from build123d import *
from build123d.topology import SkipClean

# Parameters (mm, degrees)
SKETCH_1_R               = 25
EXTRUDE_1_DEPTH          = 8
SKETCH_2_R               = 3
EXTRUDE_2_DEPTH          = 10
EXTRUDE_START            = 10
SKETCH_3_R               = 25
SKETCH_3_R_2             = 20
EXTRUDE_3_DEPTH          = 10
SKETCH_4_R               = 5
EXTRUDE_4_DEPTH          = 2
SKETCH_5_R               = 2.5
EXTRUDE_5_DEPTH          = 8
EXTRUDE_START_2          = 5
SKETCH_6_R               = 25
SKETCH_6_R_2             = 5
EXTRUDE_6_DEPTH          = 5
CUT_EXTRUDE_1_DEPTH      = 40.67366885
CUT_EXTRUDE_1_DEPTH_BACK = 40.67366885
SKETCH_8_R               = 3
SKETCH_9_R               = 5
SKETCH_9_R_2             = 3
EXTRUDE_7_DEPTH          = 6
SKETCH_10_R              = 5
EXTRUDE_8_DEPTH          = 5
SKETCH_11_R              = 3
CUT_EXTRUDE_2_DEPTH      = 5
FILLET_1_R               = 0.5


with BuildPart() as part:
    # 草图1 → 凸台-拉伸1 (new body)
    with BuildSketch(Plane.XY):
        Circle(SKETCH_1_R)
    extrude(amount=EXTRUDE_1_DEPTH)

    # 草图2 → 凸台-拉伸2 (add)
    with BuildSketch(Plane.XY.offset(8)):
        Circle(SKETCH_2_R)
    extrude(amount=EXTRUDE_2_DEPTH)

    # 草图3 → 凸台-拉伸3 (add)
    with BuildSketch(Plane(origin=(0, 0, 0), x_dir=(-1, 0, 0), z_dir=(0, 0, -1)).offset(EXTRUDE_START)):
        Circle(SKETCH_3_R)
        Circle(SKETCH_3_R_2, mode=Mode.SUBTRACT)
    extrude(amount=-EXTRUDE_3_DEPTH)

    # 草图4 → 凸台-拉伸4 (add)
    with BuildSketch(Plane(origin=(0, 0, 0), x_dir=(-1, 0, 0), z_dir=(0, 0, -1))):
        with Locations(Location((0, 0, 0), (0, 0, 180))):
            Circle(SKETCH_4_R)
    extrude(amount=EXTRUDE_4_DEPTH)

    # 草图5 → 凸台-拉伸5 (add)
    with BuildSketch(Plane(origin=(0, 0, -2), x_dir=(-1, 0, 0), z_dir=(0, 0, -1))):
        Circle(SKETCH_5_R)
    extrude(amount=EXTRUDE_5_DEPTH)

    # 草图6 → 凸台-拉伸6 (add)
    with BuildSketch(Plane(origin=(0, 0, -10), x_dir=(-1, 0, 0), z_dir=(0, 0, -1)).offset(EXTRUDE_START_2)):
        Circle(SKETCH_6_R)
        with Locations(Location((0, 0, 0), (0, 0, 180))):
            Circle(SKETCH_6_R_2, mode=Mode.SUBTRACT)
    extrude(amount=-EXTRUDE_6_DEPTH)

    # 草图8 → 切除-拉伸1 (cut, two sides: drawn at the far end of the back side and taken through both)
    with BuildSketch(Plane(origin=(0, 0, 0), x_dir=(0, 0, -1), z_dir=(1, 0, 0)).offset(-CUT_EXTRUDE_1_DEPTH_BACK)):
        with Locations(Location((6, 12.6, 0), (0, 0, 180))):
            Circle(SKETCH_8_R)
    extrude(amount=CUT_EXTRUDE_1_DEPTH + CUT_EXTRUDE_1_DEPTH_BACK, mode=Mode.SUBTRACT)

    # 草图9 → 凸台-拉伸7 (add, through all)
    with SkipClean():  # the faces are left unmerged after this step: merging them gives an invalid solid
        with BuildSketch(Plane(origin=(-19, 0, 0), x_dir=(0, 0, -1), z_dir=(1, 0, 0))):
            with Locations((6, 12.6)):
                Circle(SKETCH_9_R)
            with Locations(Location((6, 12.6, 0), (0, 0, 180))):
                Circle(SKETCH_9_R_2, mode=Mode.SUBTRACT)
        extrude(amount=-EXTRUDE_7_DEPTH)

    # 草图10 → 凸台-拉伸8 (add)
    with BuildSketch(Plane(origin=(19, 0, 0), x_dir=(0, 0, -1), z_dir=(1, 0, 0)).offset(EXTRUDE_START_2)):
        with Locations((6, 12.6)):
            Circle(SKETCH_10_R)
    extrude(amount=-EXTRUDE_8_DEPTH)

    # 草图11 → 切除-拉伸2 (cut)
    with BuildSketch(Plane(origin=(24, 0, 0), x_dir=(0, 0, -1), z_dir=(1, 0, 0))):
        with Locations(Location((6, 12.6, 0), (0, 0, 180))):
            Circle(SKETCH_11_R)
    extrude(amount=-CUT_EXTRUDE_2_DEPTH, mode=Mode.SUBTRACT)

    # 圆角1
    fillet_1_edges = [part.edges().sort_by_distance(p)[0] for p in [
        (25, 0, -15),
        (-25, 0, 8),
    ]]
    fillet(fillet_1_edges, radius=FILLET_1_R)


solid = part.part
Geometry check sheet. Reference: the model listing, model coordinates, mm. A direction names the side the tool comes from. Coordinates: 2 decimals unless noted, no trailing zeros. Write each loop counter-clockwise with the first axis right and the second up, starting at its lowest first coordinate (ties: lowest second). Pieces come first, ordered by that corner, then holes. Notation, with made-up numbers: (31.25, 21) -> (82.25, 21) arc R12 ccw to (82.25, 26) -> close; hole circle Ø2 at (78.5, 18). An arc over 180 degrees is marked (long way). One line per question, with ' | ' between items.
1. Cross-section at C-C on z = -6.5. Record the cut outline in (x, y).
Answers:
outline: (-25, 7.63) -> (-23.81, 7.63) arc R25 ccw (long way) to (23.81, 7.63) -> (24, 7.63) -> (24, 9.64) -> (17.52, 9.64) arc R20 cw (long way) to (-17.52, 9.64) -> (-25, 9.64) -> close; (-25, 15.56) -> (-12.57, 15.56) arc R20 cw to (12.57, 15.56) -> (24, 15.56) -> (24, 17.57) -> (19, 17.57) -> (19, 16.25) arc R25 ccw to (-19, 16.25) -> (-19, 17.57) -> (-25, 17.57) -> close; circle Ø5 at (0, 0)
2. Cross-section at A-A on y = 0. Record the cut outline in (x, z).
Answers:
outline: (-25, -14.5) arc R0.5 ccw to (-24.5, -15) -> (-5, -15) -> (-5, -10) -> (-20, -10) -> (-20, 0) -> (-5, 0) -> (-5, -2) -> (-2.5, -2) -> (-2.5, -10) -> (2.5, -10) -> (2.5, -2) -> (5, -2) -> (5, 0) -> (20, 0) -> (20, -10) -> (5, -10) -> (5, -15) -> (24.5, -15) arc R0.5 ccw to (25, -14.5) -> (25, 7.5) arc R0.5 ccw to (24.5, 8) -> (3, 8) -> (3, 18) -> (-3, 18) -> (-3, 8) -> (-24.5, 8) arc R0.5 ccw to (-25, 7.5) -> close
3. Cross-section at D-D on z = 6. Record the cut outline in (x, y), and give its area (3 significant figures).
Answers:
outline: circle Ø50 at (0, 0) | area: 1,960 mm²
4. Draft check along Y on faces 5 (the flat face through (0, 0, 18)), 6 (the cylindrical face through (-22.625, 17.557, -5.349)), 7 (the cylindrical face through (-3, 0, 13)). Enter one of: +Y half, -Y half, draft (parallel to the pull), parting line (faces both ways), or undercut.
Answers:
face 5: draft | face 6: undercut | face 7: parting line
5. Set-up check for faces 1 (the flat face through (-4, -4, -10)), 2 (the cylindrical face through (0.54, -2.44, -5.94)), 3 (the flat face through (0, 6, -15)), 4 (the flat face through (24, 10, -8)): record each of +Z, -Z, +X, -X, +Y, -Y from which the full face is reachable in a straight line by a thin tool's end or side.
Answers:
face 1: none | face 2: -Z | face 3: -Z, +X, -X, +Y, -Y | face 4: +Z, -Z, +X, +Y
6. Depth check by flat-ended pin: pin 1 Ø7 at (y, z) = (12.6, -6) entering from +X; pin 2 Ø8 at (x, z) = (14.5, 1.5) entering from +Y; pin 3 Ø5 at (x, z) = (-11, 3.5) entering from +Y. Enter the tip coordinate at first touch or a pass-through.
Answers:
pin 1: stops at x = 24 | pin 2: stops at y = 22.69 | pin 3: stops at y = 23.51
7. Thickness scan on probe 1 along Y at (x, z) = (0, -7); probe 2 along Y at (x, z) = (0, -12); probe 3 along Z at (x, y) = (-8, -9.5). Record the ranges inside material, lowest first. Write a range as from..to.
Answers:
probe 1: y = -25..-20, -2.5..2.5, 20..25 | probe 2: y = -25..-5, 5..25 | probe 3: z = -15..-10, 0..8
